The model under review builds one solid part; all positions refer to its coordinate system, in mm. Face numbers are marked on the shaded views. A direction names the side the tool comes from. Round coordinates to 2 decimals unless told otherwise and drop trailing zeros. Loops run counter-clockwise (first coordinate to the right, second up) from the corner with the lowest first, then second, coordinate; pieces in that order, holes last. Notation, with made-up numbers: (42, 78.25) -> (72, 78.25) arc R13 ccw to (72, 96.25) -> close; hole circle Ø5 at (22.5, 72). An arc over 180 degrees is marked (long way). Write each question's results on one line, items separated by ' | '. Start each with the question number.
Item 1: We need section D-D (y = -16). Give the boundary of the cut face in (x, z), and give its area (3 significant figures).
Item 2: We need section B-B (x = 0). Give the boundary of the cut face in (y, z) (3 decimals), and give its area (3 significant figures).
Item 3: Tool access review of the marked faces 4, 5 and 6: name each direction out of +Z, -Z, +X, -X, +Y, -Y from which nothing blocks a thin tool from reaching the whole face with its end or side.
Item 4: We need section C-C (y = -9). Give the boundary of the cut face in (x, z), and give its area (3 significant figures).
Item 5: For L1, parallel to X at y = -20, z = 0; L2, parallel to X at y = -6, z = -1.25; L3, parallel to X at y = -5.8, z = 0 (3 decimals), list the stretches that pass through material, from the lowest coordinate up. Write a range as from..to.
Item 6: We need section A-A (z = 0). Give the boundary of the cut face in (x, y) (3 decimals), and give its area (3 significant figures).
Item 7: Clearance check with flat-ended pins moving along their axes: pin 1 Ø2 at (y, z) = (-18.5, -7) entering from -X; pin 2 Ø4 at (x, z) = (6, -6.5) entering from +Y; pin 3 Ø2 at (x, z) = (8, -5) entering from -Y; pin 4 Ø5 at (y, z) = (6, 7) entering from +X. State where each tip first meets the part, or that it passes through.
Item 8: Mouldability with a two-part tool opening along X and no side actions: class the marked faces 1, 2 and 3 as pulls with the +X half, pulls with the -X half, needs draft (parallel to the pull), parting line crosses it, or undercut.
from build123d import *

# Parameters (mm, degrees)
SKETCH1_R                = 3
BOSS_EXTRUDE1_DEPTH      = 10
SKETCH2_R                = 4.775
BOSS_EXTRUDE2_DEPTH      = 10.35
BOSS_EXTRUDE3_DEPTH      = 3
BOSS_EXTRUDE3_DEPTH_BACK = 3
SKETCH3_R                = 9.5
SKETCH4_R                = 12.4
SKETCH4_R_2              = 9.5
BOSS_EXTRUDE4_DEPTH      = 9.35
BOSS_EXTRUDE5_START      = 8.8
SKETCH5_R                = 12.4
SKETCH5_R_2              = 9.5
BOSS_EXTRUDE5_DEPTH      = 8.8


with BuildPart() as part:
    # Sketch1 → Boss-Extrude1 (new body)
    with BuildSketch(Plane(origin=(0, 0, 0), x_dir=(1, 0, 0), z_dir=(0, 1, 0))):
        with Locations(Location((0, 0, 0), (0, 0, 270))):
            Circle(SKETCH1_R)
    extrude(amount=BOSS_EXTRUDE1_DEPTH)

    # Sketch2 → Boss-Extrude2 (add)
    with BuildSketch(Plane.XZ):
        with Locations(Location((0, 0, 0), (0, 0, 270))):
            Circle(SKETCH2_R)
    extrude(amount=BOSS_EXTRUDE2_DEPTH)

    # Sketch3 → Boss-Extrude3 (add, two sides: drawn at the far end of the back side and taken through both)
    with BuildSketch(Plane.XZ.offset(10.35).offset(-BOSS_EXTRUDE3_DEPTH_BACK)):
        with Locations(Location((0, 0, 0), (0, 0, 270))):
            Circle(SKETCH3_R)
    extrude(amount=BOSS_EXTRUDE3_DEPTH + BOSS_EXTRUDE3_DEPTH_BACK)

    # Sketch4 → Boss-Extrude4 (add)
    with BuildSketch(Plane.XZ.offset(13.35)):
        with Locations(Location((0, 0, 0), (0, 0, 270))):
            Circle(SKETCH4_R)
        with Locations(Location((0, 0, 0), (0, 0, 270))):
            Circle(SKETCH4_R_2, mode=Mode.SUBTRACT)
    extrude(amount=-BOSS_EXTRUDE4_DEPTH)

    # Sketch5 → Boss-Extrude5 (add)
    with BuildSketch(Plane.XZ.offset(13.35).offset(BOSS_EXTRUDE5_START)):
        with Locations(Location((0, 0, 0), (0, 0, 270))):
            Circle(SKETCH5_R)
        with Locations(Location((0, 0, 0), (0, 0, 270))):
            Circle(SKETCH5_R_2, mode=Mode.SUBTRACT)
    extrude(amount=-BOSS_EXTRUDE5_DEPTH)


solid = part.part
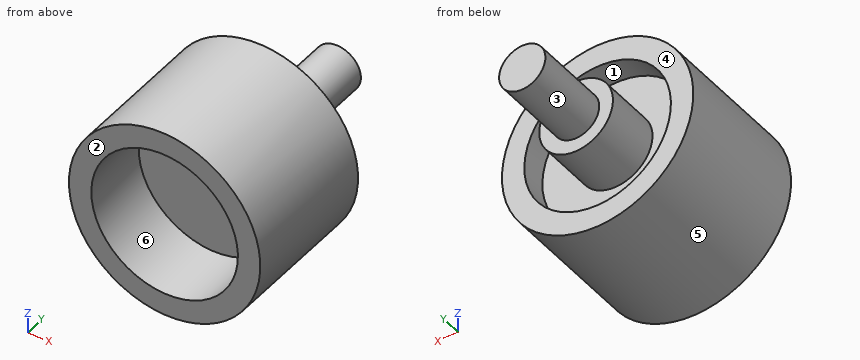
Here are the results:
1) outline: circle Ø24.8 at (0, 0); hole circle Ø19 at (0, 0) | area: 200 mm2
2) outline: (-22.15, -12.4) -> (-4, -12.4) -> (-4, -9.5) -> (-7.35, -9.5) -> (-7.35, -4.775) -> (0, -4.775) -> (0, -3) -> (10, -3) -> (10, 3) -> (0, 3) -> (0, 4.775) -> (-7.35, 4.775) -> (-7.35, 9.5) -> (-4, 9.5) -> (-4, 12.4) -> (-22.15, 12.4) -> (-22.15, 9.5) -> (-13.35, 9.5) -> (-13.35, -9.5) -> (-22.15, -9.5) -> close | area: 349 mm2
3) face 4: +Y | face 5: +Y, -Y | face 6: -Y
4) outline: circle Ø24.8 at (0, 0) | area: 483 mm2
5) L1: x = -12.4..-9.5, 9.5..12.4 | L2: x = -12.34..-9.42, -4.61..4.61, 9.42..12.34 | L3: x = -12.4..-9.5, -4.775..4.775, 9.5..12.4
6) outline: (-12.4, -22.15) -> (-9.5, -22.15) -> (-9.5, -13.35) -> (9.5, -13.35) -> (9.5, -22.15) -> (12.4, -22.15) -> (12.4, -4) -> (9.5, -4) -> (9.5, -7.35) -> (4.775, -7.35) -> (4.775, 0) -> (3, 0) -> (3, 10) -> (-3, 10) -> (-3, 0) -> (-4.775, 0) -> (-4.775, -7.35) -> (-9.5, -7.35) -> (-9.5, -4) -> (-12.4, -4) -> close | area: 349 mm2
7) pin 1: stops at x = -10.85 | pin 2: stops at y = -4 | pin 3: stops at y = -22.15 | pin 4: passes through
8) face 1: undercut | face 2: needs draft | face 3: parting line crosses it
